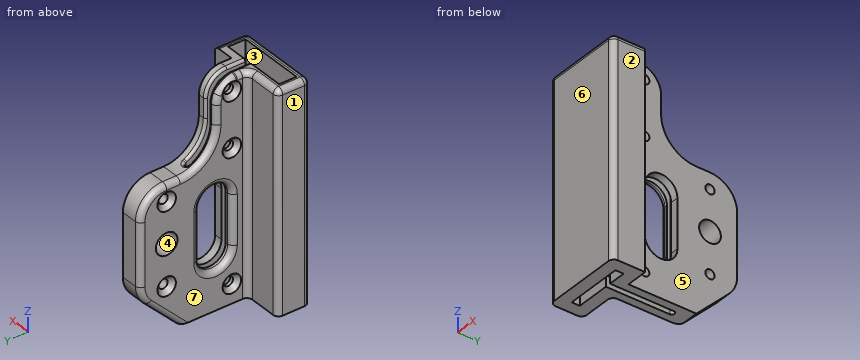
from build123d import *

# Parameters (mm, degrees)
PAD_DEPTH       = 80
POCKET_DEPTH    = 76
SKETCH002_R     = 1.7
SKETCH002_R_2   = 4
POCKET001_DEPTH = 16.001
POCKET002_DEPTH = 5
POCKET003_DEPTH = 22.001
CHAMFER_SIZE    = 15
FILLET_R        = 10
FILLET001_R     = 10
FILLET002_R     = 8
FILLET003_R     = 8
CHAMFER001_SIZE = 1.7
CHAMFER002_SIZE = 1.7
CHAMFER003_SIZE = 1.7
CHAMFER004_SIZE = 1.7
CHAMFER005_SIZE = 1.7
FILLET004_R     = 2
FILLET005_R     = 2
FILLET006_R     = 2
FILLET007_R     = 2
FILLET008_R     = 2
FILLET009_R     = 2
FILLET010_R     = 0.9
FILLET011_R     = 0.9
FILLET012_R     = 0.9


with BuildPart() as part:
    # Sketch → Pad (new body)
    with BuildSketch(Plane.XY):
        Polygon((-4, 0), (-4, 40), (4, 40), (4, 18), (4, 0), (12, 0), (12, -12), (-18, -12), (-18, 0), align=None)
    extrude(amount=PAD_DEPTH)

    # Sketch001 → Pocket (cut)
    with BuildSketch(Plane.XY.offset(80)):
        Polygon((1, -2.8), (1, 20), (-1, 20), (-1, -2.8), (-15.25, -2.8), (-15.25, -9.2), (9.25, -9.2), (9.25, -2.8), align=None)
    extrude(amount=-POCKET_DEPTH, mode=Mode.SUBTRACT)

    # Sketch002 → Pocket001 (cut, through all)
    with BuildSketch(Plane(origin=(-4, 0, 0), x_dir=(0, -1, 0), z_dir=(-1, 0, 0))):
        with Locations((-6, 7)):
            Circle(SKETCH002_R)
        with Locations((-6, 55)):
            Circle(SKETCH002_R)
        with Locations((-6, 75)):
            Circle(SKETCH002_R)
        with Locations((-30, 46)):
            Circle(SKETCH002_R)
        with Locations((-30, 16)):
            Circle(SKETCH002_R)
        with Locations((-30, 31)):
            Circle(SKETCH002_R_2)
    extrude(amount=-POCKET001_DEPTH, mode=Mode.SUBTRACT)

    # Sketch003 → Pocket002 (cut)
    with BuildSketch(Plane(origin=(0, 0, 0), x_dir=(1, 0, 0), z_dir=(0, 0, -1))):
        Polygon((-13.5, 7.5), (7.5, 7.5), (7.5, 4.5), (1, 4.5), (1, -20), (-1, -20), (-1, 4.5), (-13.5, 4.5), align=None)
    extrude(amount=-POCKET002_DEPTH, mode=Mode.SUBTRACT)

    # Sketch004 → Pocket003 (cut, through all)
    with BuildSketch(Plane.YZ.offset(4)):
        with BuildLine():
            Line((12, 85), (45, 85))
            Line((45, 85), (45, 52))
            Line((45, 52), (25, 52))
            ThreePointArc((12, 65), (15.807612, 55.807612), (25, 52))
            Line((12, 65), (12, 85))
        make_face()
        with BuildLine():
            ThreePointArc((18, 38), (12, 44), (6, 38))
            Line((6, 38), (6, 20))
            ThreePointArc((6, 20), (12, 14), (18, 20))
            Line((18, 38), (18, 20))
        make_face()
    extrude(amount=-POCKET003_DEPTH, mode=Mode.SUBTRACT)

    # Chamfer
    chamfer_edges = [part.edges().sort_by_distance(p)[0] for p in [
        (0, 40, 0),
    ]]
    chamfer(chamfer_edges, length=CHAMFER_SIZE)

    # Fillet
    fillet_edges = [part.edges().sort_by_distance(p)[0] for p in [
        (0, 40, 15),
    ]]
    fillet(fillet_edges, radius=FILLET_R)

    # Fillet001
    fillet001_edges = [part.edges().sort_by_distance(p)[0] for p in [
        (0, 40, 52),
    ]]
    fillet(fillet001_edges, radius=FILLET001_R)

    # Fillet002
    fillet002_edges = [part.edges().sort_by_distance(p)[0] for p in [
        (-2.5, 12, 80),
    ]]
    fillet(fillet002_edges, radius=FILLET002_R)

    # Fillet003
    fillet003_edges = [part.edges().sort_by_distance(p)[0] for p in [
        (2.5, 12, 80),
    ]]
    fillet(fillet003_edges, radius=FILLET003_R)

    # Chamfer001
    chamfer001_edges = [part.edges().sort_by_distance(p)[0] for p in [
        (-4, 7.7, 75),
    ]]
    chamfer(chamfer001_edges, length=CHAMFER001_SIZE)

    # Chamfer002
    chamfer002_edges = [part.edges().sort_by_distance(p)[0] for p in [
        (-4, 7.7, 55),
    ]]
    chamfer(chamfer002_edges, length=CHAMFER002_SIZE)

    # Chamfer003
    chamfer003_edges = [part.edges().sort_by_distance(p)[0] for p in [
        (-4, 31.7, 46),
    ]]
    chamfer(chamfer003_edges, length=CHAMFER003_SIZE)

    # Chamfer004
    chamfer004_edges = [part.edges().sort_by_distance(p)[0] for p in [
        (-4, 31.7, 16),
    ]]
    chamfer(chamfer004_edges, length=CHAMFER004_SIZE)

    # Chamfer005
    chamfer005_edges = [part.edges().sort_by_distance(p)[0] for p in [
        (-4, 7.7, 7),
    ]]
    chamfer(chamfer005_edges, length=CHAMFER005_SIZE)

    # Fillet004
    fillet004_edges = [part.edges().sort_by_distance(p)[0] for p in [
        (-4, 0, 40),
    ]]
    fillet(fillet004_edges, radius=FILLET004_R)

    # Fillet005
    fillet005_edges = [part.edges().sort_by_distance(p)[0] for p in [
        (-18, 0, 40),
    ]]
    fillet(fillet005_edges, radius=FILLET005_R)

    # Fillet006
    fillet006_edges = [part.edges().sort_by_distance(p)[0] for p in [
        (-18, -12, 40),
    ]]
    fillet(fillet006_edges, radius=FILLET006_R)

    # Fillet007
    fillet007_edges = [part.edges().sort_by_distance(p)[0] for p in [
        (12, -12, 40),
    ]]
    fillet(fillet007_edges, radius=FILLET007_R)

    # Fillet008
    fillet008_edges = [part.edges().sort_by_distance(p)[0] for p in [
        (-4, 40, 30.571068),
    ]]
    fillet(fillet008_edges, radius=FILLET008_R)

    # Fillet009
    fillet009_edges = [part.edges().sort_by_distance(p)[0] for p in [
        (-4, 18, 29),
    ]]
    fillet(fillet009_edges, radius=FILLET009_R)

    # Fillet010
    fillet010_edges = [part.edges().sort_by_distance(p)[0] for p in [
        (-1, 20, 29),
    ]]
    fillet(fillet010_edges, radius=FILLET010_R)

    # Fillet011
    fillet011_edges = [part.edges().sort_by_distance(p)[0] for p in [
        (1, 20, 29),
    ]]
    fillet(fillet011_edges, radius=FILLET011_R)

    # Fillet012
    fillet012_edges = [part.edges().sort_by_distance(p)[0] for p in [
        (1, 0.6, 80),
    ]]
    fillet(fillet012_edges, radius=FILLET012_R)


solid = part.part
Model file for the job. Use its own axes, mm. Face numbers are marked on the shaded views. A direction names the side the tool comes from. Give positions to 0.01 mm unless a question says otherwise; leave off trailing zeros. Order: outer loops, then holes, each group sorted by start corner. A loop starts at its lowest first (then second) coordinate and runs counter-clockwise, first axis right, second up. Notation, with made-up numbers: (49.5, 65.25) -> (59.5, 65.25) arc R22 ccw to (59.5, 93.25) -> close; hole circle Ø2 at (41.25, -29.5). An arc over 180 degrees is marked (long way). Use CSV: the item, a comma, the result in double quotes.
1. Band-saw the part on B-B, the plane y = -5.5. Give the cut face in (x, z).
Outcome:
outline,"(-18, 0) -> (-13.5, 0) -> (-13.5, 4) -> (-15.25, 4) -> (-15.25, 80) -> (-16, 80) arc R2 ccw to (-18, 78) -> close; (7.5, 0) -> (12, 0) -> (12, 78) arc R2 ccw to (10, 80) -> (9.25, 80) -> (9.25, 4) -> (7.5, 4) -> close"
2. Band-saw the part on C-C, the plane z = 68.5. Give the cut face in (x, y), then the cut area to 3 significant figures.
Outcome:
outline,"(-18, -10) arc R2 ccw to (-16, -12) -> (10, -12) arc R2 ccw to (12, -10) -> (12, 0) -> (4, 0) -> (4, 12) -> (1.9, 12) arc R0.9 ccw to (1, 11.1) -> (1, -2.8) -> (9.25, -2.8) -> (9.25, -9.2) -> (-15.25, -9.2) -> (-15.25, -2.8) -> (-1, -2.8) -> (-1, 11.1) arc R0.9 ccw to (-1.9, 12) -> (-2, 12) arc R2 ccw to (-4, 10) -> (-4, 2) arc R2 cw to (-6, 0) -> (-16, 0) arc R2 ccw to (-18, -2) -> close"
area,"267 mm²"
3. Mould opens along X. For the marked faces 1, 2, 3 and 4 say: +X half, -X half, draft (parallel to the pull), parting line (faces both ways), or undercut.
Outcome:
face 1,"-X half"
face 2,"+X half"
face 3,"undercut"
face 4,"draft"
4. 3-axis set-ups, long thin cutter, end or side, ignore diameter. For the marked faces 5, 6 and 7: which of +Z, -Z, +X, -X, +Y, -Y reach the whole face in a straight line?
Outcome:
face 5,"+Z, -Z, +X, +Y"
face 6,"+Z, -Z, +X, -X, -Y"
face 7,"+Z, -Z, -X, +Y"
5. Drop flat-ended pins along their axis: pin 1 (3 mm diameter, centred on y = 3.5, z = 44.5, fed in from +X); pin 2 (5.5 mm diameter, centred on y = 6, z = 75, fed in from -X); pin 3 (4 mm diameter, centred on x = 2.5, y = 26.5, fed in from +Z). Give the stop position or say it passes through.
Outcome:
pin 1,"x = 4"
pin 2,"x = -3.35"
pin 3,"z = 52.01"
6. Band-saw the part on D-D, the plane y = 16. Count the separate pieces of the cut face and the enclosed holes in it, then the cut area to 3 significant figures.
Outcome:
separate pieces,"4"
enclosed holes,"0"
area,"168 mm²"
7. Band-saw the part on A-A, the plane x = -8. Give the cut face in (y, z), then the cut area to 3 significant figures.
Outcome:
outline,"(-12, 0) -> (-7.5, 0) -> (-7.5, 4) -> (-9.2, 4) -> (-9.2, 80) -> (-10, 80) arc R2 ccw to (-12, 78) -> close; (-4.5, 0) -> (0, 0) -> (0, 78) arc R2 ccw to (-2, 80) -> (-2.8, 80) -> (-2.8, 4) -> (-4.5, 4) -> close"
area,"460 mm²"
8. Drill centre lines: line 1 along X through (y, z) = (3.5, 9.5); line 2 along X through (y, z) = (-8.5, 50); line 3 along Y through (x, z) = (7, 6). Where is each one in solid material? Low to high. Write a range as from..to.
Outcome:
line 1,"-4..-1, 1..4"
line 2,"-18..-15.25, 9.25..12"
line 3,"-12..-9.2, -2.8..0"
